Work out the finished part from the listing and answer in its coordinate system (mm). Round coordinates to 2 decimals unless told otherwise and drop trailing zeros. Order: outer loops, then holes, each group sorted by start corner. A loop starts at its lowest first (then second) coordinate and runs counter-clockwise, first axis right, second up. Notation, with made-up numbers: (-21, 39) - (18, 39) arc R20 ccw to (18, 76) - close; hole circle Ø10 at (-39, -15). An arc over 180 degrees is marked (long way). Answer in a Markdown table with one row per item.
from build123d import *

# Parameters (mm, degrees)
SKETCH1_W                  = 863.6
SKETCH1_H                  = 50.8
BOSS_EXTRUDE2_DEPTH        = 50.8
F_1_2_0_5_DIAMETER_HOLE1_D = 12.7


with BuildPart() as part:
    # Sketch1 → Boss-Extrude2 (new body)
    with BuildSketch(Plane(origin=(0, 0, 0), x_dir=(1, 0, 0), z_dir=(0, 1, 0))):
        with BuildLine():
            Line((-431.8, -25.4), (-431.8, 25.4))
            ThreePointArc((-431.8, 25.4), (-457.2, 0), (-431.8, -25.4))
        make_face()
        Rectangle(SKETCH1_W, SKETCH1_H)
        with BuildLine():
            ThreePointArc((431.8, 25.4), (457.2, 0), (431.8, -25.4))
            Line((431.8, -25.4), (431.8, 25.4))
        make_face()
    extrude(amount=BOSS_EXTRUDE2_DEPTH)

    # 1/2 (0.5) Diameter Hole1 (through all)
    with Locations(Plane(origin=(0, 50.8, 0), x_dir=(1, 0, 0), z_dir=(0, 1, 0))):
        with Locations((431.8, 0), (-431.8, 0)):
            Hole(F_1_2_0_5_DIAMETER_HOLE1_D / 2)


solid = part.part
1) Each of these flat-tipped pins is pushed along its axis until it touches: pin 1 (2 mm diameter, centred on y = 38, z = -14.5, fed in from +X); pin 2 (3 mm diameter, centred on y = 41, z = 1.5, fed in from -X); pin 3 (12 mm diameter, centred on y = 45, z = 13, fed in from +X). Where does it stop, or does it pass through?
Filled in:
| item | result |
|---|---|
| pin 1 | stops at x = 453.32 |
| pin 2 | stops at x = -457.2 |
| pin 3 | stops at x = 456.22 |
2) Find the intervals of material crossed by probe 1 along Z at (x, y) = (-431.8, 37); probe 2 along X at (y, z) = (39, -5); probe 3 along X at (y, z) = (34, -4), in increasing order. Write a range as from..to.
Filled in:
| item | result |
|---|---|
| probe 1 | z = -25.4..-6.35, 6.35..25.4 |
| probe 2 | x = -456.7..-435.71, -427.89..427.89, 435.71..456.7 |
| probe 3 | x = -456.88..-436.73, -426.87..426.87, 436.73..456.88 |
3) Find section A-A, the plane y = 42.5. Give the vertices of the cut face in (x, z).
Filled in:
| item | result |
|---|---|
| outline | (-431.8, -25.4) - (431.8, -25.4) arc R25.4 ccw to (431.8, 25.4) - (-431.8, 25.4) arc R25.4 ccw to start; hole circle Ø12.7 at (-431.8, 0); hole circle Ø12.7 at (431.8, 0) |
